Work out the finished part from the listing and answer in its coordinate system (mm). Give positions to 0.01 mm unless a question says otherwise; leave off trailing zeros.
```python
from build123d import *

# Parameters (mm, degrees)
BOSS_EXTRUDE1_DEPTH = 6.35


with BuildPart() as part:
    # Sketch1 → Boss-Extrude1 (new body)
    with BuildSketch(Plane(origin=(0, 0, 0), x_dir=(1, 0, 0), z_dir=(0, 1, 0))):
        with BuildLine():
            Line((60.8717096, 62.8883934), (60.8717096, 62.8914922))
            add(Edge.make_bspline(
                [(60.8717096, 62.8914922), (59.8243914, 63.663195), (58.7701898, 64.0421376), (57.4679572, 64.1179312)],
                knots=[0, 0, 0, 0, 1, 1, 1, 1], degree=3))
            add(Edge.make_bspline(
                [(57.4679572, 64.1179312), (56.2483762, 64.1799326), (55.035704, 64.1029452), (53.8230318, 64.0879338)],
                knots=[0, 0, 0, 0, 1, 1, 1, 1], degree=3))
            add(Edge.make_bspline(
                [(53.8230318, 64.0879338), (51.390804, 64.0629402), (48.9585508, 64.0379212), (46.526323, 64.018922)],
                knots=[0, 0, 0, 0, 1, 1, 1, 1], degree=3))
            add(Edge.make_bspline(
                [(46.526323, 64.018922), (41.661842, 63.963931), (36.797361, 63.9154424), (31.9329054, 63.8674364)],
                knots=[0, 0, 0, 0, 1, 1, 1, 1], degree=3))
            add(Edge.make_bspline(
                [(31.9329054, 63.8674364), (29.4937688, 63.837439), (27.061541, 63.8174238), (24.6292878, 63.7914396)],
                knots=[0, 0, 0, 0, 1, 1, 1, 1], degree=3))
            add(Edge.make_bspline(
                [(24.6292878, 63.7914396), (23.4097322, 63.7764282), (22.19706, 63.7714244), (20.9775044, 63.7564384)],
                knots=[0, 0, 0, 0, 1, 1, 1, 1], degree=3))
            add(Edge.make_bspline(
                [(20.9775044, 63.7564384), (19.7579234, 63.741427), (18.5590434, 63.8389376), (17.3463712, 63.5084328)],
                knots=[0, 0, 0, 0, 1, 1, 1, 1], degree=3))
            add(Edge.make_bspline(
                [(17.3463712, 63.5084328), (13.8599164, 62.5575838), (8.5751416, 56.1841396), (6.8250308, 53.6141422)],
                knots=[0, 0, 0, 0, 1, 1, 1, 1], degree=3))
            add(Edge.make_bspline(
                [(6.8250308, 53.6141422), (-4.716018, 36.6573308), (-0.7610602, 13.6096756), (15.7754066, 1.469136)],
                knots=[0, 0, 0, 0, 1, 1, 1, 1], degree=3))
            add(Edge.make_bspline(
                [(15.7754066, 1.469136), (16.8296082, 0.6974332), (17.876901, 0.3184906), (19.1860424, 0.2495804)],
                knots=[0, 0, 0, 0, 1, 1, 1, 1], degree=3))
            add(Edge.make_bspline(
                [(19.1860424, 0.2495804), (20.3987146, 0.180594), (21.6113868, 0.2545842), (22.8309424, 0.2695956)],
                knots=[0, 0, 0, 0, 1, 1, 1, 1], degree=3))
            add(Edge.make_bspline(
                [(22.8309424, 0.2695956), (25.2563122, 0.2945892), (27.6954234, 0.3195828), (30.1276766, 0.3455924)],
                knots=[0, 0, 0, 0, 1, 1, 1, 1], degree=3))
            add(Edge.make_bspline(
                [(30.1276766, 0.3455924), (34.9921322, 0.3955796), (39.8566132, 0.442087), (44.7210942, 0.490093)],
                knots=[0, 0, 0, 0, 1, 1, 1, 1], degree=3))
            add(Edge.make_bspline(
                [(44.7210942, 0.490093), (47.153322, 0.5200904), (49.5855752, 0.5400802), (52.0246864, 0.5660898)],
                knots=[0, 0, 0, 0, 1, 1, 1, 1], degree=3))
            add(Edge.make_bspline(
                [(52.0246864, 0.5660898), (53.2373586, 0.5810758), (54.4569396, 0.5960872), (55.6696118, 0.601091)],
                knots=[0, 0, 0, 0, 1, 1, 1, 1], degree=3))
            add(Edge.make_bspline(
                [(55.6696118, 0.601091), (56.8891674, 0.616077), (58.0880474, 0.5185918), (59.3076284, 0.8490712)],
                knots=[0, 0, 0, 0, 1, 1, 1, 1], degree=3))
            add(Edge.make_bspline(
                [(59.3076284, 0.8490712), (62.7940578, 1.7999456), (68.0788326, 8.1802732), (69.8220346, 10.7433872)],
                knots=[0, 0, 0, 0, 1, 1, 1, 1], degree=3))
            add(Edge.make_bspline(
                [(69.8220346, 10.7433872), (81.3631088, 27.7001732), (77.408151, 50.7478792), (60.8717096, 62.8883934)],
                knots=[0, 0, 0, 0, 1, 1, 1, 1], degree=3))
        make_face()
        with BuildLine():
            add(Edge.make_bspline(
                [(59.5970106, 32.3954902), (59.6175084, 30.121733), (61.4849164, 28.2889452), (63.7655824, 28.3164788)],
                knots=[0, 0, 0, 0, 1, 1, 1, 1], degree=3))
            add(Edge.make_bspline(
                [(63.7655824, 28.3164788), (66.046223, 28.336494), (67.8721274, 30.2043846), (67.8514772, 32.485076)],
                knots=[0, 0, 0, 0, 1, 1, 1, 1], degree=3))
            add(Edge.make_bspline(
                [(67.8514772, 32.485076), (67.830954, 34.7588332), (65.963546, 36.591621), (63.6829054, 36.5709454)],
                knots=[0, 0, 0, 0, 1, 1, 1, 1], degree=3))
            add(Edge.make_bspline(
                [(63.6829054, 36.5709454), (61.4022394, 36.5409226), (59.5694516, 34.6761308), (59.5970106, 32.3954902)],
                knots=[0, 0, 0, 0, 1, 1, 1, 1], degree=3))
        make_face(mode=Mode.SUBTRACT)
        with BuildLine():
            add(Edge.make_bspline(
                [(17.0569636, 31.9682876), (17.0776138, 29.6876216), (15.2448514, 27.8203914), (12.9710942, 27.7997412)],
                knots=[0, 0, 0, 0, 1, 1, 1, 1], degree=3))
            add(Edge.make_bspline(
                [(12.9710942, 27.7997412), (10.6904282, 27.7747222), (8.823198, 29.6049954), (8.8025224, 31.885636)],
                knots=[0, 0, 0, 0, 1, 1, 1, 1], degree=3))
            add(Edge.make_bspline(
                [(8.8025224, 31.885636), (8.7749634, 34.1593932), (10.6077512, 36.0266234), (12.8884172, 36.0541824)],
                knots=[0, 0, 0, 0, 1, 1, 1, 1], degree=3))
            add(Edge.make_bspline(
                [(12.8884172, 36.0541824), (15.1621744, 36.0741722), (17.0294046, 34.2489282), (17.0569636, 31.9682876)],
                knots=[0, 0, 0, 0, 1, 1, 1, 1], degree=3))
        make_face(mode=Mode.SUBTRACT)
    extrude(amount=BOSS_EXTRUDE1_DEPTH)


solid = part.part
```
Q1. Consider line 1 along X through (y, z) = (5.5, -31); line 2 along X through (y, z) = (5.75, -35.5); line 3 along Z through (x, y) = (22, 1.25). Determine where each line is inside the solid, lowest interval first.
Q2. Given pin 1 (1 mm diameter, centred on x = 11, z = -32, fed in from +Y); pin 2 (3 mm diameter, centred on y = 3, z = -38.5, fed in from +X); pin 3 (3 mm diameter, centred on y = 2, z = -10.5, fed in from +X); pin 4 (1.5 mm diameter, centred on x = 14, y = 5.5, fed in from -Z), each flat-ended and moving along its own axis, determine where each tip first touches the part or whether it passes through.
Q3. Section A-A on y = 2 is taken. State how many separate pieces and enclosed holes the cut face has, plus the area to 3 significant figures.
Check result:
1. line 1: x = 0.24 to 8.91, 16.95 to 59.85, 67.59 to 76.41
1. line 2: x = 0.36 to 10.87, 14.99 to 60.95, 66.5 to 76.28
1. line 3: z = -63.77 to -0.25
2. pin 1: passes through
2. pin 2: stops at x = 76.12
2. pin 3: stops at x = 70.64
2. pin 4: stops at z = -62.13
3. separate pieces: 1
3. enclosed holes: 2
3. area: 4,090 mm2
